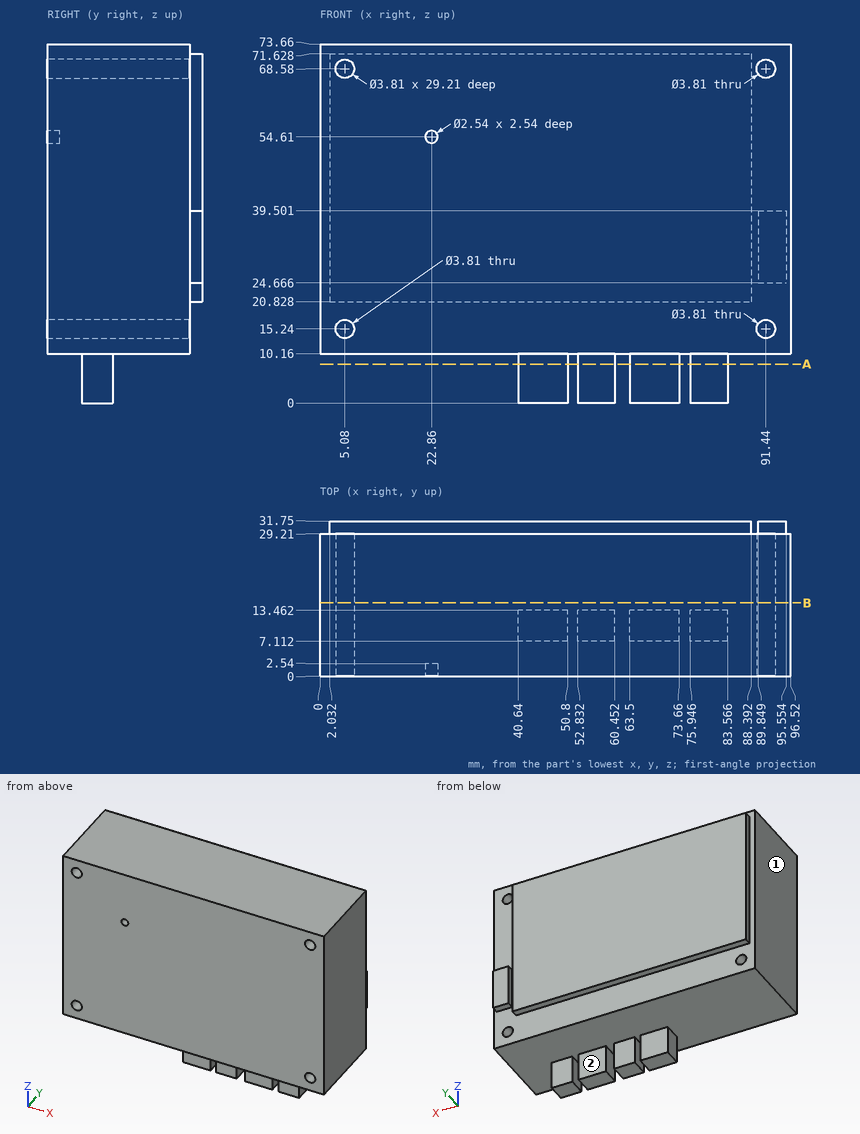
Answer from the drawing. Dimensions are ordinates in mm from the lowest x, y and z of the part. A direction names the side the tool comes from. Round coordinates to 2 decimals unless told otherwise and drop trailing zeros. Loops run counter-clockwise (first coordinate to the right, second up) from the corner with the lowest first, then second, coordinate; pieces in that order, holes last.
(1) Find the intervals of material crossed by L1, parallel to Z at x = 5.08, y = 9.75 (1 decimal); L2, parallel to X at y = 15, z = 15; L3, parallel to X at y = 8.5, z = 15.24 (1 decimal), in increasing order.
Computed values:
L1: z = 10.2 to 13.3, 17.1 to 66.7, 70.5 to 73.7
L2: x = 0 to 3.19, 6.97 to 89.55, 93.33 to 96.52
L3: x = 0 to 3.2, 7 to 89.5, 93.3 to 96.5
(2) For the marked faces 1 and 2, determine the directions among +Z, -Z, +X, -X, +Y, -Y from which every point of the face is accessible in a straight line to the end or side of a thin tool.
Computed values:
face 1: +Z, -Z, -X, +Y, -Y
face 2: -Z, +X, -X, +Y
(3) The part is cut by section B-B, the plane y = 15. Give the vertices of the cut face in (x, z) (1 decimal).
Computed values:
outline: (0, 10.2) - (96.5, 10.2) - (96.5, 73.7) - (0, 73.7) - close; hole circle Ø3.8 at (5.1, 15.2); hole circle Ø3.8 at (5.1, 68.6); hole circle Ø3.8 at (91.4, 15.2); hole circle Ø3.8 at (91.4, 68.6)
(4) The part is cut by section A-A, the plane z = 8. Give the vertices of the cut face in (x, y).
Computed values:
outline: (40.64, 7.11) - (50.8, 7.11) - (50.8, 13.46) - (40.64, 13.46) - close; (52.83, 7.11) - (60.45, 7.11) - (60.45, 13.46) - (52.83, 13.46) - close; (63.5, 7.11) - (73.66, 7.11) - (73.66, 13.46) - (63.5, 13.46) - close; (75.95, 7.11) - (83.57, 7.11) - (83.57, 13.46) - (75.95, 13.46) - close
(5) Each of these flat-tipped pins is pushed along its axis until it touches: P1, Ø1.5, axis at x = 38, y = 20.5, coming from the -Z side; P2, Ø8.5, axis at x = 58, z = 7, coming from the +Y side; P3, Ø1.3, axis at y = 31, z = 43, coming from the -X side; P4, Ø3.5, axis at x = 5.08, z = 15.24, coming from the +Y side. Where does it stop, or does it pass through?
Computed values:
P1: stops at z = 10.16
P2: stops at y = 29.21
P3: stops at x = 2.03
P4: passes through
